from build123d import *

# Parameters (mm, degrees)
F0_R     = 5.5
F0_R_2   = 2.5
F1_DEPTH = 10
F2_W     = 21
F2_H     = 21
F3_DEPTH = 4
F4_W     = 15.5
F4_H     = 15.5
F5_DEPTH = 2
F6_R     = 4
F7_R     = 1.25
F8_DEPTH = 10
F9_R     = 3


with BuildPart() as f1:
    # F0 (on Top) → F1 (new body)
    with BuildSketch(Plane.XY):
        Circle(F0_R)
        Circle(F0_R_2, mode=Mode.SUBTRACT)
    extrude(amount=F1_DEPTH)

    # F2 (on face) → F3 (join)
    with BuildSketch(Plane.XY.offset(10)):
        Rectangle(F2_W, F2_H)
    extrude(amount=F3_DEPTH)

    # F4 (on face) → F5 (cut)
    with BuildSketch(Plane.XY.offset(14)):
        Rectangle(F4_W, F4_H)
    extrude(amount=-F5_DEPTH, mode=Mode.SUBTRACT)

    # F6
    f6_edges = [f1.edges().sort_by_distance(p)[0] for p in [
        (10.5, 10.5, 12),
        (10.5, -10.5, 12),
        (-10.5, -10.5, 12),
        (-10.5, 10.5, 12),
    ]]
    fillet(f6_edges, radius=F6_R)

    # F7 (on Front) → F8 (cut)
    with BuildSketch(Plane.XZ):
        with Locations((0, 3)):
            Circle(F7_R)
    extrude(amount=-F8_DEPTH, mode=Mode.SUBTRACT)

    # F9
    f9_edges = [f1.edges().sort_by_distance(p)[0] for p in [
        (-7.75, 7.75, 13),
        (7.75, 7.75, 13),
        (-7.75, -7.75, 13),
        (7.75, -7.75, 13),
        (-5.5, 0, 10),
    ]]
    fillet(f9_edges, radius=F9_R)


solid = f1.part
Here's how the part is built. I have some questions about the finished solid (model axes, mm). A direction names the side the tool comes from. Coordinates: 2 decimals unless noted, no trailing zeros. Write each loop counter-clockwise with the first axis right and the second up, starting at its lowest first coordinate (ties: lowest second). Pieces come first, ordered by that corner, then holes.
Item 1: If I drill on line 1 (Y direction, x = -3, z = 12.75); line 2 (Z direction, x = 0, y = 3.7); line 3 (Y direction, x = 0, z = 6), over which ranges is the centre line in solid material (lowest first)?
Item 2: Will these pins go through, and if not, where does the flat tip stop? pin 1 (2 mm diameter, centred on x = 4.5, y = -2, fed in from +Z); pin 2 (2 mm diameter, centred on x = 4.5, z = 4.5, fed in from +Y); pin 3 (2 mm diameter, centred on y = 4.5, z = 8, fed in from +X).
Item 3: If we mould it in two halves opening along X, with no side actions, what happens to faces 4 (the flat face through (-7.75, 0, 13)), 5 (the flat face through (10.5, 0, 12)), 6 (the flat face through (0, 9, 10)), 7 (the flat face through (-10.5, 0, 12))? For each: +X half, -X half, draft (parallel to the pull), parting line (faces both ways), or undercut.
Item 4: I want a section at B-B on z = 5.75. Write out the boundary of the cut face in (x, y), and give its area (3 significant figures).
Item 5: I want a section at D-D on x = 9.25. Write out the boundary of the cut face in (y, z).
Item 6: On a 3-axis mill with a long thin cutter (end or side, diameter ignored), from which of +Z, -Z, +X, -X, +Y, -Y can I reach the whole of each face in a straight line? I mean faces 1 (the cylindrical face through (-1.25, 3.81, 3.05)), 2 (the flat face through (7.75, 0, 13)), 3 (the cylindrical face through (-1.19, -5.37, 3.45)). Say none if no direction works.
Item 7: I want a section at A-A on x = 0. Write out the boundary of the cut face in (y, z).
Item 8: I want a section at C-C on y = 0. Write out the boundary of the cut face in (x, z), and give its area (3 significant figures).
Findings below:
1. line 1: y = -10.5 to -7.75, 7.75 to 10.5
1. line 2: z = 0 to 1.75, 4.25 to 12
1. line 3: y = -5.5 to -2.5, 2.5 to 5.5
2. pin 1: stops at z = 12
2. pin 2: stops at y = 4.24
2. pin 3: stops at x = 4.69
3. face 4: undercut
3. face 5: +X half
3. face 6: draft
3. face 7: -X half
4. outline: circle Ø11 at (0, 0); hole circle Ø5 at (0, 0)
4. area: 75.4 mm2
5. outline: (-9.4, 10) - (9.4, 10) - (9.4, 14) - (-9.4, 14) - close
6. face 1: +Y
6. face 2: +Z
6. face 3: -Z
7. outline: (-10.5, 10) - (-8.5, 10) arc R3 cw to (-5.5, 7) - (-5.5, 0) - (-2.5, 0) - (-2.5, 10) - (2.5, 10) - (2.5, 4.25) - (5.5, 4.25) - (5.5, 7) arc R3 cw to (8.5, 10) - (10.5, 10) - (10.5, 14) - (7.75, 14) - (7.75, 12) - (-7.75, 12) - (-7.75, 14) - (-10.5, 14) - close; (2.5, 0) - (5.5, 0) - (5.5, 1.75) - (2.5, 1.75) - close
8. outline: (-10.5, 10) - (-8.5, 10) arc R3 cw to (-5.5, 7) - (-5.5, 0) - (-2.5, 0) - (-2.5, 10) - (2.5, 10) - (2.5, 0) - (5.5, 0) - (5.5, 7) arc R3 cw to (8.5, 10) - (10.5, 10) - (10.5, 14) - (7.75, 14) - (7.75, 12) - (-7.75, 12) - (-7.75, 14) - (-10.5, 14) - close
8. area: 117 mm2
